Could you check a few things on this model? Use its own coordinates, in mm. Give positions to 0.01 mm unless a question says otherwise; leave off trailing zeros. Order: outer loops, then holes, each group sorted by start corner. A loop starts at its lowest first (then second) coordinate and runs counter-clockwise, first axis right, second up. Notation, with made-up numbers: (-6.75, 7.25) - (33.25, 7.25) arc R18 cw to (33.25, 28.25) - close; hole circle Ø5 at (-4, -10.75). An arc over 180 degrees is marked (long way). Put each result on its own line as item: value.
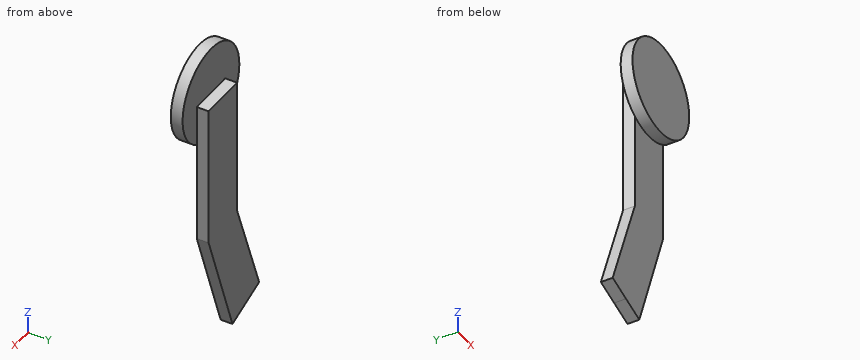
Autodesk Inventor part; units mm, degrees
ref_plane "YZ Plane" through (0, 0, 0) normal (1, 0, 0) x (0, 1, 0)
ref_plane "XZ Plane" through (0, 0, 0) normal (0, 1, 0) x (-1, 0, 0)
ref_plane "XY Plane" through (0, 0, 0) normal (0, 0, 1) x (1, 0, 0)
sketch "Sketch1" plane through (0, 0, 0) normal (0, 1, 0) x (-1, 0, 0)
  circle A0 centre (0, 0) radius 20
  dimension "d0" = 40
extrude "Extrusion1" add sketch "Sketch1" along normal blind 5
sketch "Sketch2" plane through (0, 5, 0) normal (0, 1, 0) x (1, 0, 0)
  line L0 (0, 0) -> (-10, 0)
  line L1 (-10, 0) -> (-10, 60)
  line L2 (-10, 60) -> (0, 60)
  line L3 (0, 60) -> (0, 0)
  line L4 (0, 0) -> (10, 0)
  line L5 (10, 0) -> (10, 60)
  line L6 (10, 60) -> (0, 60)
  line L7 (0, 60) -> (0, 0)
  line L8 (0, 60) -> (-16.246, 104.6354)
  line L9 (0, 60) -> (-9.3969, 56.5798)
  line L10 (-9.3969, 56.5798) -> (-25.6429, 101.2152)
  line L11 (-25.6429, 101.2152) -> (-16.246, 104.6354)
  line L12 (-16.246, 104.6354) -> (-6.849, 108.0556)
  line L13 (-6.849, 108.0556) -> (10, 60)
  dimension "d3" = 10
  dimension "d4" = 60
  dimension "d5" = 10
  dimension "d7" = 47.5
  dimension "d8" = 160
  dimension "d9" = 10
  dimension "d10" = 10
extrude "Extrusion2" add sketch "Sketch2" along normal blind 5
properties part number "scale_r_arm"
1) If I drill on line 1 (Y direction, x = 17, z = -5.5); line 2 (Y direction, x = -2.5, z = -54.5); line 3 (X direction, y = 9, z = -4.5), over which ranges is the centre line in solid material (lowest first)? Write a range as [from, to].
Filled in:
line 1: y = [0, 5]
line 2: y = [5, 10]
line 3: x = [-10, 10]
2) I'm going to push flat-ended pins straight in: pin 1 (3 mm diameter, centred on x = -13, z = -9, fed in from +Y); pin 2 (4 mm diameter, centred on x = -9.5, y = 4.5, fed in from -Z); pin 3 (6 mm diameter, centred on y = 2.5, z = -45, fed in from -X); pin 4 (2 mm diameter, centred on y = 3.5, z = -34, fed in from -X). Where does each tip first touch, or does it pass through?
Filled in:
pin 1: stops at y = 5
pin 2: stops at z = -107.8
pin 3: stops at x = -10
pin 4: passes through
3) Suppose I cut it at B-B, the plane x = 0. List the corners of the cut face in (y, z) for me.
Filled in:
outline: (0, -20) - (5, -20) - (5, -88.52) - (10, -88.52) - (10, 0) - (5, 0) - (5, 20) - (0, 20) - close
4) Suppose I cut it at A-A, the plane y = 7. List the corners of the cut face in (x, z) for me.
Filled in:
outline: (-25.64, -101.22) - (-16.25, -104.64) - (-6.85, -108.06) - (10, -60) - (10, 0) - (-10, 0) - (-10, -58.24) - close
5) Suppose I cut it at D-D, the plane x = 8.5. List the corners of the cut face in (y, z) for me.
Filled in:
outline: (0, -18.1) - (5, -18.1) - (5, -64.28) - (10, -64.28) - (10, 0) - (5, 0) - (5, 18.1) - (0, 18.1) - close
6) Suppose I cut it at C-C, the plane z = -49. List the corners of the cut face in (x, y) for me.
Filled in:
outline: (-10, 5) - (10, 5) - (10, 10) - (-10, 10) - close
